from build123d import *

# Parameters (mm, degrees)
F1_DEPTH = 31.75
F3_DEPTH = 25.401
F5_DEPTH = 12.7
F7_DEPTH = 12.7


# Not quite as in the source:
# - a length typed as a fraction of an inch, garbled in the dataset ("3 / 203.2 mm" for 3/8 in), is restored


with BuildPart() as f1:
    # F0 (on Top) → F1 (new body)
    with BuildSketch(Plane.XY):
        Polygon((-25.4, 38.1), (-44.45, 38.1), (-44.45, 0), (-25.4, 0), (-25.4, 12.7), (0, 12.7), (0, 25.4), (-25.4, 25.4), align=None)
    extrude(amount=F1_DEPTH)

    # F2 (on face) → F3 (cut, through all)
    with BuildSketch(Plane.XZ.offset(-12.7)):
        Polygon((0, 31.75), (-12.7, 31.75), (0, 0), align=None)
    extrude(amount=-F3_DEPTH, mode=Mode.SUBTRACT)

    # F4 (on face) → F5 (join)
    with BuildSketch(Plane.XZ.offset(-12.7)):
        Polygon((-12.7, 0), (-25.4, 31.75), (-25.4, 0), align=None)
    extrude(amount=F5_DEPTH)

    # F6 (on face) → F7 (join)
    with BuildSketch(Plane(origin=(0, 25.4, 0), x_dir=(-1, 0, 0), z_dir=(0, 1, 0))):
        Polygon((25.4, 0), (25.4, 31.75), (12.7, 0), align=None)
    extrude(amount=F7_DEPTH)


solid = f1.part
Geometry check sheet. Reference: the model listing, model coordinates, mm. A direction names the side the tool comes from. Give positions to 0.01 mm unless a question says otherwise; leave off trailing zeros. Write each loop counter-clockwise with the first axis right and the second up, starting at its lowest first coordinate (ties: lowest second). Pieces come first, ordered by that corner, then holes.
1) Go/stop test with flat-tipped pins: pin 1 Ø12 at (y, z) = (24.5, 13.5) entering from +X; pin 2 Ø8 at (x, z) = (-18, 27) entering from -Y; pin 3 Ø6 at (x, z) = (-8, 6.5) entering from +Y; pin 4 Ø6 at (x, y) = (-7, 30) entering from -Z. Record where each tip stops, or that it passes through.
Values follow:
pin 1: stops at x = -3
pin 2: stops at y = 12.7
pin 3: stops at y = 25.4
pin 4: passes through
2) Cross-section at A-A (z = 5). Record the boundary of the cut face in (x, y).
Values follow:
outline: (-44.45, 0) - (-14.7, 0) - (-14.7, 12.7) - (-2, 12.7) - (-2, 25.4) - (-14.7, 25.4) - (-14.7, 38.1) - (-44.45, 38.1) - close
3) Thickness scan on line 1 (Y direction, x = -11.5, z = 3); line 2 (X direction, y = 6, z = 6); line 3 (X direction, y = 7, z = 24). Record the ranges inside material, lowest first.
Values follow:
line 1: y = 12.7 to 25.4
line 2: x = -44.45 to -15.1
line 3: x = -44.45 to -22.3
4) Cross-section at C-C (y = 35). Record the boundary of the cut face in (x, z), plus the area to 3 significant figures.
Values follow:
outline: (-44.45, 0) - (-12.7, 0) - (-25.4, 31.75) - (-44.45, 31.75) - close
area: 806 mm2
5) Set-up check for faces 1 (the face through (-6.44, 18.96, 16.1)), 2 (the face through (-13, 25.4, 16)), 3 (the face through (-18.96, 6.44, 15.65)): record each of +Z, -Z, +X, -X, +Y, -Y from which the full face is reachable in a straight line by a thin tool's end or side.
Values follow:
face 1: +Z, +X, +Y, -Y
face 2: +Z, +X, +Y
face 3: +Z, +X, -Y
6) Cross-section at B-B (x = -15.5). Record the boundary of the cut face in (y, z).
Values follow:
outline: (0, 0) - (38.1, 0) - (38.1, 7) - (25.4, 7) - (25.4, 31.75) - (12.7, 31.75) - (12.7, 7) - (0, 7) - close
7) Cross-section at D-D (x = -6.5). Record the boundary of the cut face in (y, z), plus the area to 3 significant figures.
Values follow:
outline: (12.7, 0) - (25.4, 0) - (25.4, 16.25) - (12.7, 16.25) - close
area: 206 mm2
